Build history of the part. All positions in model axes, mm. A direction names the side the tool comes from. Round coordinates to 2 decimals unless told otherwise and drop trailing zeros. Order: outer loops, then holes, each group sorted by start corner. A loop starts at its lowest first (then second) coordinate and runs counter-clockwise, first axis right, second up. Notation, with made-up numbers: (-30.5, 26) -> (-21.5, 26) arc R25 cw to (-21.5, 52) -> close; hole circle Ø2 at (88, 68). An arc over 180 degrees is marked (long way). Write item = value, one per line.
from build123d import *

# Parameters (mm, degrees)
SKETCH_1_W                  = 25
SKETCH_1_H                  = 25
EXTRUDE_1_DEPTH             = 25
SKETCH_2_W                  = 23
SKETCH_2_H                  = 23
CUT_EXTRUDE_1_DEPTH         = 44.301270189
HOLE_WIZARD_2_0_2_1_D       = 2
HOLE_WIZARD_2_1_2_1_1_D     = 2.1
HOLE_WIZARD_2_1_2_1_1_DEPTH = 25
FILLET_1_R                  = 3


with BuildPart() as part:
    # 草图1 → 凸台-拉伸1 (new body)
    with BuildSketch(Plane.XY.offset(25)):
        with Locations((-12.5, 12.5)):
            Rectangle(SKETCH_1_W, SKETCH_1_H)
    extrude(amount=-EXTRUDE_1_DEPTH)

    # 草图2 → 切除-拉伸1 (cut, through all)
    with BuildSketch(Plane.XZ):
        with Locations((-13.5, 13.5)):
            Rectangle(SKETCH_2_W, SKETCH_2_H)
    extrude(amount=-CUT_EXTRUDE_1_DEPTH, mode=Mode.SUBTRACT)

    # Ø2.0 (2) 直径孔1 (through all)
    with Locations(Plane.XY.offset(2)):
        with Locations((-10, 20), (-10, 6), (-20, 6), (-20, 19.98825417)):
            Hole(HOLE_WIZARD_2_0_2_1_D / 2)

    # Ø2.1 (2.1) 直径孔1
    with Locations(Plane(origin=(0, 0, 0), x_dir=(0, 0, -1), z_dir=(1, 0, 0))):
        with Locations((-19, 20.5), (-19, 4.5), (-19, 12.5), (-11, 4.5), (-11, 20.5)):
            Hole(HOLE_WIZARD_2_1_2_1_1_D / 2, depth=HOLE_WIZARD_2_1_2_1_1_DEPTH)

    # 圆角1
    fillet_1_edges = [part.edges().sort_by_distance(p)[0] for p in [
        (-2, 12.5, 2),
    ]]
    fillet(fillet_1_edges, radius=FILLET_1_R)


solid = part.part
Q1. Which spindle directions (+Z, -Z, +X, -X, +Y, -Y) get a long thin tool onto all of the face, cutting with end or side? Do faces 5 (the face through (-25, 12, 1)), 6 (the face through (-2, 12, 15)). Say none if no direction does.
Check values:
face_5 = +Z, -Z, -X, +Y, -Y
face_6 = +Z, -X, +Y, -Y
Q2. Cut at D-D, the plane y = 12.5. List the corners of the cut face in (x, z).
Check values:
outline = (-25, 0) -> (0, 0) -> (0, 17.95) -> (-2, 17.95) -> (-2, 5) arc R3 cw to (-5, 2) -> (-25, 2) -> close; (-2, 20.05) -> (0, 20.05) -> (0, 25) -> (-2, 25) -> close
Q3. Cut at A-A, the plane y = 6. List the corners of the cut face in (x, z), and give its area (3 significant figures).
Check values:
outline = (-25, 0) -> (-21, 0) -> (-21, 2) -> (-25, 2) -> close; (-19, 0) -> (-11, 0) -> (-11, 2) -> (-19, 2) -> close; (-9, 0) -> (0, 0) -> (0, 25) -> (-2, 25) -> (-2, 5) arc R3 cw to (-5, 2) -> (-9, 2) -> close
area = 89.9 mm²
Q4. Probe probe 1 along Y at (x, z) = (-20, 1.15); probe 2 along Y at (x, z) = (-1.1, 11); probe 3 along Y at (x, z) = (-1.4, 19). List the from-to ranges inside material, lowest first.
Check values:
probe_1 = 0 to 5, 7 to 18.99, 20.99 to 25
probe_2 = 0 to 3.45, 5.55 to 19.45, 21.55 to 25
probe_3 = 0 to 3.45, 5.55 to 11.45, 13.55 to 19.45, 21.55 to 25
Q5. Cut at B-B, the plane x = -10. List the corners of the cut face in (y, z).
Check values:
outline = (0, 0) -> (5, 0) -> (5, 2) -> (0, 2) -> close; (7, 0) -> (19, 0) -> (19, 2) -> (7, 2) -> close; (21, 0) -> (25, 0) -> (25, 2) -> (21, 2) -> close
Q6. Flat gauge pins, fed straight in: pin 1 (3.5 mm diameter, centred on y = 12.5, z = 19, fed in from -X); pin 2 (12 mm diameter, centred on x = -9.5, z = 9, fed in from -Y); pin 3 (10 mm diameter, centred on x = -19, y = 14, fed in from +Z). Where does each tip first touch, or does it go through?
Check values:
pin_1 = -2
pin_2 = through
pin_3 = 2
Q7. Mould opens along Z. For faces 1 (the face through (-2.9, 12.68, 2.86)), 2 (the face through (-10, 7, 1)), 3 (the face through (-1.01, 19.86, 18.17)), 4 (the face through (-1.01, 4.82, 12)) say: released by +Z, released by -Z, zero draft, split by the parting line, or undercut.
Check values:
face_1 = released by +Z
face_2 = zero draft
face_3 = undercut
face_4 = undercut
Q8. Cut at C-C, the plane z = 19. List the corners of the cut face in (x, y).
Check values:
outline = (-2, 0) -> (0, 0) -> (0, 3.45) -> (-2, 3.45) -> close; (-2, 5.55) -> (0, 5.55) -> (0, 11.45) -> (-2, 11.45) -> close; (-2, 13.55) -> (0, 13.55) -> (0, 19.45) -> (-2, 19.45) -> close; (-2, 21.55) -> (0, 21.55) -> (0, 25) -> (-2, 25) -> close
